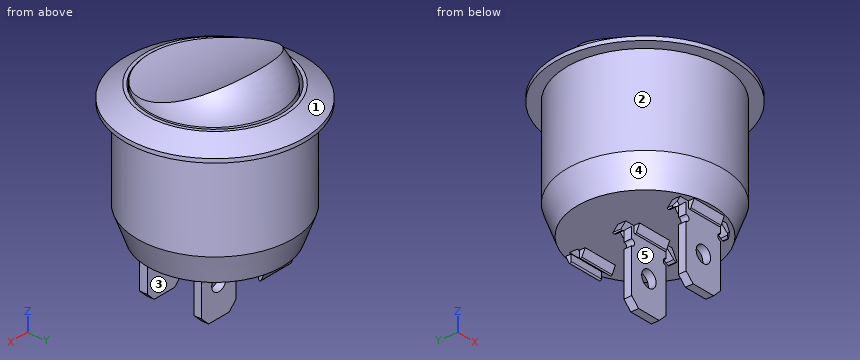
```python
from build123d import *

# Parameters (mm, degrees)
SKETCH1_R                = 10
BOSS_EXTRUDE1_DEPTH      = 15
SKETCH2_R                = 11.5
BOSS_EXTRUDE2_DEPTH      = 2
SKETCH3_R                = 8.5
CUT_EXTRUDE1_DEPTH       = 2
CUT_EXTRUDE2_REACH       = 17
SKETCH4_R                = 8.5
SKETCH4_R_2              = 7
SKETCH5_R                = 10
SKETCH5_W                = 5
SKETCH5_H                = 1
BOSS_EXTRUDE3_DEPTH      = 0.1
BOSS_EXTRUDE3_DEPTH_BACK = 1
SKETCH6_W                = 5
SKETCH6_H                = 1
BOSS_EXTRUDE4_DEPTH      = 9
SKETCH7_R                = 8.25
BOSS_EXTRUDE5_DEPTH      = 6
CUT_EXTRUDE3_DEPTH       = 16
CUT_EXTRUDE3_DEPTH_BACK  = 16
SKETCH10_R               = 1.05
SKETCH10_R_2             = 0.4
CUT_EXTRUDE4_DEPTH       = 13
CHAMFER1_SIZE            = 1
CHAMFER2_SIZE            = 1
BOSS_EXTRUDE8_DEPTH      = 1
BOSS_EXTRUDE9_DEPTH      = 2.2
CHAMFER4_SIZE            = 1.5
CHAMFER4_SIZE2           = 2.598076211


with BuildPart() as part:
    # Sketch1 → Boss-Extrude1 (new body)
    with BuildSketch(Plane.XY):
        Circle(SKETCH1_R)
    extrude(amount=BOSS_EXTRUDE1_DEPTH)

    # Sketch2 → Boss-Extrude2 (add)
    with BuildSketch(Plane.XY.offset(15)):
        Circle(SKETCH2_R)
    extrude(amount=BOSS_EXTRUDE2_DEPTH)

    # Sketch3 → Cut-Extrude1 (cut)
    with BuildSketch(Plane.XY.offset(17)):
        Circle(SKETCH3_R)
    extrude(amount=-CUT_EXTRUDE1_DEPTH, mode=Mode.SUBTRACT)

    # Sketch4 → Cut-Extrude2 (cut, up to next)
    with BuildSketch(Plane.XY.offset(15), mode=Mode.PRIVATE) as cut_extrude2_sk1:
        Circle(SKETCH4_R)
        Circle(SKETCH4_R_2, mode=Mode.SUBTRACT)
    cut_extrude2_tool1 = extrude(cut_extrude2_sk1.sketch, amount=-CUT_EXTRUDE2_REACH, mode=Mode.PRIVATE) & part.part
    add(cut_extrude2_tool1.solids().sort_by_distance((-8.259584, 0, 15))[0], mode=Mode.SUBTRACT)

    # Sketch5 → Boss-Extrude3 (add, two sides)
    with BuildSketch(Plane(origin=(0, 0, 0), x_dir=(-1, 0, 0), z_dir=(0, 0, -1))) as boss_extrude3_sk:
        Circle(SKETCH5_R)
        with Locations((0, 7)):
            Rectangle(SKETCH5_W, SKETCH5_H, mode=Mode.SUBTRACT)
    extrude(amount=BOSS_EXTRUDE3_DEPTH)
    extrude(boss_extrude3_sk.sketch, amount=-BOSS_EXTRUDE3_DEPTH_BACK)

    # Sketch6 → Boss-Extrude4 (add)
    with BuildSketch(Plane(origin=(0, 0, -0.1), x_dir=(-1, 0, 0), z_dir=(0, 0, -1))):
        with Locations((0, -7)):
            Rectangle(SKETCH6_W, SKETCH6_H)
        Rectangle(SKETCH6_W, SKETCH6_H)
    extrude(amount=BOSS_EXTRUDE4_DEPTH)

    # Sketch7 → Boss-Extrude5 (add)
    with BuildSketch(Plane.XY.offset(15)):
        with Locations((0, -0.15)):
            Circle(SKETCH7_R)
    extrude(amount=BOSS_EXTRUDE5_DEPTH)

    # Sketch8 → Cut-Revolve1 (revolve, cut)
    with BuildSketch(Plane(origin=(0, 0, 0), x_dir=(0, 0, -1), z_dir=(1, 0, 0))):
        with BuildLine():
            Line((-17, 8.1), (-21.761349269, 8.1))
            Line((-21.761349269, 8.1), (-21.761349269, 5.797413216))
            Line((-21.761349269, 5.797413216), (-21, 5.797413216))
            ThreePointArc((-21, 5.797413216), (-19.162388314, 7.230803795), (-17, 8.1))
        make_face()
    revolve(axis=Axis((0, -0.15, 21), (0, 0, 1)), mode=Mode.SUBTRACT)

    # Sketch9 → Cut-Extrude3 (cut, two sides)
    with BuildSketch(Plane(origin=(0, 0, 0), x_dir=(0, 0, -1), z_dir=(1, 0, 0))) as cut_extrude3_sk:
        with BuildLine():
            Line((-21, 5.797413216), (-21, -8.374651695))
            Line((-21, -8.374651695), (-17.1, -8.374651695))
            ThreePointArc((-17.1, -8.374651695), (-18.085767141, -1.023272716), (-21, 5.797413216))
        make_face()
    extrude(amount=CUT_EXTRUDE3_DEPTH, mode=Mode.SUBTRACT)
    extrude(cut_extrude3_sk.sketch, amount=-CUT_EXTRUDE3_DEPTH_BACK, mode=Mode.SUBTRACT)

    # Sketch10 → Cut-Extrude4 (cut, through all)
    with BuildSketch(Plane(origin=(0, 0.5, 0), x_dir=(1, 0, 0), z_dir=(0, 1, 0))):
        with Locations((0, 5.1)):
            Circle(SKETCH10_R)
        with Locations((-2.5, 2.1)):
            Circle(SKETCH10_R_2)
        with Locations((2.5, 2.1)):
            Circle(SKETCH10_R_2)
    extrude(amount=-CUT_EXTRUDE4_DEPTH, mode=Mode.SUBTRACT)

    # Chamfer1
    chamfer1_edges = [part.edges().sort_by_distance(p)[0] for p in [
        (2.5, 0, -9.1),
        (-2.5, 0, -9.1),
    ]]
    chamfer(chamfer1_edges, length=CHAMFER1_SIZE)

    # Chamfer2
    chamfer2_edges = [part.edges().sort_by_distance(p)[0] for p in [
        (-2.5, -7, -9.1),
        (2.5, -7, -9.1),
    ]]
    chamfer(chamfer2_edges, length=CHAMFER2_SIZE)

    # Sketch11 → Boss-Extrude8 (add)
    with BuildSketch(Plane(origin=(0, 0.5, 0), x_dir=(1, 0, 0), z_dir=(0, 1, 0))):
        with BuildLine():
            Line((-3.629263342, 1.290449142), (-2.5, 0.318466995))
            Line((-2.5, 0.318466995), (-2.5, 0.1))
            Line((-2.5, 0.1), (-3.382092802, 0.1))
            Line((-3.382092802, 0.1), (-4.076192043, 1.304590563))
            ThreePointArc((-4.076192043, 1.304590563), (-4.0626874, 1.422710807), (-3.945800247, 1.444440068))
            Line((-3.945800247, 1.444440068), (-3.629263342, 1.290449142))
        make_face()
        with BuildLine():
            Line((2.5, 0.318466995), (2.5, 0.1))
            Line((2.5, 0.1), (3.382092802, 0.1))
            Line((3.382092802, 0.1), (4.076192043, 1.304590563))
            ThreePointArc((4.076192043, 1.304590563), (4.0626874, 1.422710807), (3.945800247, 1.444440068))
            Line((3.945800247, 1.444440068), (3.629263342, 1.290449142))
            Line((3.629263342, 1.290449142), (2.5, 0.318466995))
        make_face()
    boss_extrude8 = extrude(amount=-BOSS_EXTRUDE8_DEPTH)

    # Sketch12 → Boss-Extrude9 (add, symmetric)
    with BuildSketch(Plane(origin=(0, 0, 0), x_dir=(0, 0, -1), z_dir=(1, 0, 0))):
        with BuildLine():
            Line((0.1, 0.55), (0.935536489, 0.55))
            ThreePointArc((0.935536489, 0.55), (1.08205668, 0.667877829), (0.998290443, 0.836242215))
            Line((0.998290443, 0.836242215), (0.1, 1.25))
            Line((0.1, 1.25), (0.1, 0.55))
        make_face()
        with BuildLine():
            Line((0.1, -1.25), (0.1, -0.55))
            Line((0.1, -0.55), (0.935536489, -0.55))
            ThreePointArc((0.935536489, -0.55), (1.08205668, -0.667877829), (0.998290443, -0.836242215))
            Line((0.998290443, -0.836242215), (0.1, -1.25))
        make_face()
    boss_extrude9 = extrude(amount=BOSS_EXTRUDE9_DEPTH, both=True)

    # Mirror4: Boss-Extrude8, Boss-Extrude9 across plane
    add(boss_extrude8.mirror(Plane.ZX.offset(-3.5)))
    add(boss_extrude9.mirror(Plane.ZX.offset(-3.5)))

    # Mirror5: Boss-Extrude9 across plane
    add(boss_extrude9.mirror(Plane.ZX.offset(3.5)))

    # Sketch13 → Cut-Revolve2 (revolve, cut)
    with BuildSketch(Plane(origin=(0, 0, 0), x_dir=(0, 0, -1), z_dir=(1, 0, 0))):
        Polygon((1.764077397, 8.06685955), (-3.547182339, 10), (0.1, 10), (1.764077397, 10), align=None)
    revolve(axis=Axis((0, 0, 0), (0, 0, -1)), mode=Mode.SUBTRACT)

    # Chamfer4
    chamfer4_edges = [part.edges().sort_by_distance(p)[0] for p in [
        (-11.5, 0, 17),
    ]]
    chamfer4_side = [part.faces().sort_by_distance(p)[0] for p in [
        (-11.5, 0, 16),
    ]]
    chamfer(chamfer4_edges, length=CHAMFER4_SIZE, length2=CHAMFER4_SIZE2, reference=chamfer4_side[0])


solid = part.part
```
Can you work these out from the model? Positions are in its coordinate system, mm. Face numbers are marked on the shaded views. A direction names the side the tool comes from. Coordinates: 2 decimals unless noted, no trailing zeros. Loops run counter-clockwise (first coordinate to the right, second up) from the corner with the lowest first, then second, coordinate; pieces in that order, holes last. Notation, with made-up numbers: (33, -3.75) - (49, -3.75) arc R23 cw to (49, 4.25) - close; hole circle Ø10 at (-5, -36.5). An arc over 180 degrees is marked (long way). Use a Markdown table: item, result.
Item 1: Will these pins go through, and if not, where does the flat tip stop? pin 1 (10 mm diameter, centred on x = 9, y = -8.5, fed in from +Z); pin 2 (6 mm diameter, centred on y = -2, z = 7.5, fed in from +X); pin 3 (2 mm diameter, centred on x = 0, z = 12.5, fed in from -Y); pin 4 (1.3 mm diameter, centred on x = 0, z = -5.1, fed in from +Y).
Numbers:
| item | result |
|---|---|
| pin 1 | stops at z = 17.47 |
| pin 2 | stops at x = 10 |
| pin 3 | stops at y = -10 |
| pin 4 | passes through |
Item 2: I want a section at A-A on z = -5.1. Please give me the cut outline in (x, y), and give its area (3 significant figures).
Numbers:
| item | result |
|---|---|
| outline | (-2.5, -7.5) - (-1.05, -7.5) - (-1.05, -6.5) - (-2.5, -6.5) - close; (-2.5, -0.5) - (-1.05, -0.5) - (-1.05, 0.5) - (-2.5, 0.5) - close; (1.05, -7.5) - (2.5, -7.5) - (2.5, -6.5) - (1.05, -6.5) - close; (1.05, -0.5) - (2.5, -0.5) - (2.5, 0.5) - (1.05, 0.5) - close |
| area | 5.80 mm2 |
Item 3: I want a section at C-C on x = 0. Give the number of separate pieces and of enclosed holes in the cut face, and give its area (3 significant figures).
Numbers:
| item | result |
|---|---|
| separate pieces | 4 |
| enclosed holes | 0 |
| area | 337 mm2 |
Item 4: If I drill on probe 1 along Y at (x, z) = (0, 9.75); probe 2 along X at (y, z) = (-7, -5.1); probe 3 along Y at (x, z) = (-6, 13.5), over which ranges is the centre line in solid material (lowest first)? Write a range as from..to.
Numbers:
| item | result |
|---|---|
| probe 1 | y = -10..-8.5, -7..7, 8.5..10 |
| probe 2 | x = -2.5..-1.05, 1.05..2.5 |
| probe 3 | y = -8..-6.02, -3.61..3.61, 6.02..8 |
Item 5: We'd pull the mould along Y, two halves only. Please class the marked faces 3, 4 and 5: released by +Y, released by -Y, zero draft, split by the parting line, or undercut.
Numbers:
| item | result |
|---|---|
| face 3 | undercut |
| face 4 | split by the parting line |
| face 5 | undercut |
Item 6: For the marked faces 1 and 2, which set-ups out of +Z, -Z, +X, -X, +Y, -Y let a thin tool reach every point of the face, with its end or its side?
Numbers:
| item | result |
|---|---|
| face 1 | +Z |
| face 2 | -Z |
Item 7: I want a section at B-B on z = 5. Please give me the cut outline in (x, y).
Numbers:
| item | result |
|---|---|
| outline | circle Ø20 at (0, 0); circle Ø14 at (0, 0); hole circle Ø17 at (0, 0) |
